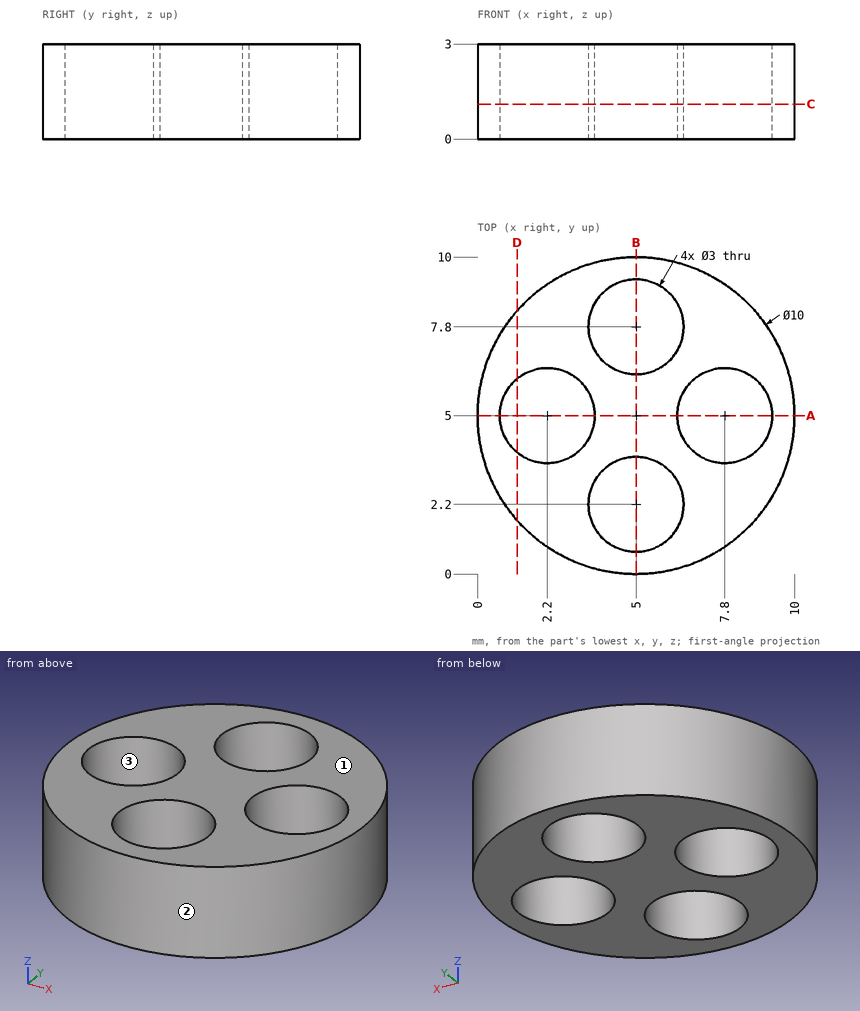
Can you work these out from the drawing? Everything is in mm from the part's minimum corner. Coordinates: 2 decimals unless noted, no trailing zeros. Order: outer loops, then holes, each group sorted by start corner. A loop starts at its lowest first (then second) coordinate and runs counter-clockwise, first axis right, second up. Notation, with made-up numbers: (-29.75, -24) -> (23.25, -24) arc R18 ccw to (23.25, 9) -> close; hole circle Ø7 at (-33, 31). An arc over 180 degrees is marked (long way). Return JSON: item names as keys, results as strings.
1) If we section it at A-A on y = 5: List the corners of the cut face in (x, z) for me.
Conclusion:
{"outline": "(0, 0) -> (0.7, 0) -> (0.7, 3) -> (0, 3) -> close; (3.7, 0) -> (6.3, 0) -> (6.3, 3) -> (3.7, 3) -> close; (9.3, 0) -> (10, 0) -> (10, 3) -> (9.3, 3) -> close"}
2) Thinking about a two-plate mould opening in X: for the marked faces 1, 2 and 3, which applies, +X half, -X half, draft (parallel to the pull), parting line (faces both ways), or undercut?
Conclusion:
{"face 1": "draft", "face 2": "parting line", "face 3": "undercut"}
3) I'm going to push a flat-ended pin straight in: P1, Ø1.8, axis at x = 2.2, y = 5, coming from the -Z side. Where does the tip first touch, or does it pass through?
Conclusion:
{"P1": "passes through"}
4) If we section it at C-C on z = 1.1: List the corners of the cut face in (x, y) for me, plus the area to 3 significant figures.
Conclusion:
{"outline": "circle Ø10 at (5, 5); hole circle Ø3 at (2.2, 5); hole circle Ø3 at (5, 2.2); hole circle Ø3 at (5, 7.8); hole circle Ø3 at (7.8, 5)", "area": "50.3 mm²"}
5) If we section it at D-D on x = 1.25: List the corners of the cut face in (y, z) for me.
Conclusion:
{"outline": "(1.69, 0) -> (3.84, 0) -> (3.84, 3) -> (1.69, 3) -> close; (6.16, 0) -> (8.31, 0) -> (8.31, 3) -> (6.16, 3) -> close"}
6) If I drill on probe 1 along Y at (x, z) = (5, 1.9); probe 2 along Y at (x, z) = (3.75, 0.9), over which ranges is the centre line in solid material (lowest first)?
Conclusion:
{"probe 1": "y = 0 to 0.7, 3.7 to 6.3, 9.3 to 10", "probe 2": "y = 0.16 to 1.37, 3.03 to 6.97, 8.63 to 9.84"}
